For this review, take the finished solid that the model builds, in its own axes (mm). Face numbers are marked on the shaded views. A direction names the side the tool comes from. Coordinates: 2 decimals unless noted, no trailing zeros. Loops run counter-clockwise (first coordinate to the right, second up) from the corner with the lowest first, then second, coordinate; pieces in that order, holes last. Notation, with made-up numbers: (79.25, 87) -> (110.25, 87) arc R7 cw to (110.25, 95) -> close; hole circle Ø4 at (-7.75, -11.5). An arc over 180 degrees is marked (long way). One line per item, written item: value.
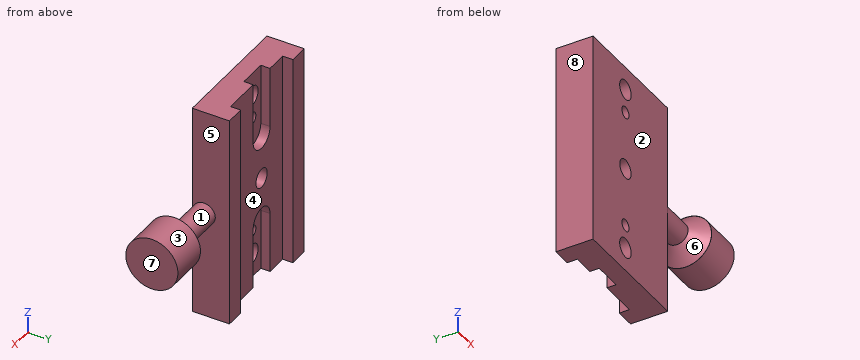
from build123d import *

# Parameters (mm, degrees)
BOSS_EXTRUDE1_DEPTH = 90
SKETCH2_R           = 4.75
BOSS_EXTRUDE2_DEPTH = 37
SKETCH3_R           = 11
BOSS_EXTRUDE3_DEPTH = 16
CHAMFER1_SIZE       = 6.2
SKETCH4_R           = 4
SKETCH4_R_2         = 2.5
SKETCH4_R_3         = 4.1
CUT_EXTRUDE1_DEPTH  = 16.97152885
CUT_EXTRUDE2_DEPTH  = 3.9


with BuildPart() as part:
    # Sketch1 → Boss-Extrude1 (new body)
    with BuildSketch(Plane.XY):
        Polygon((0, 0), (30, 0), (30, 15.7), (22, 15.7), (22, 11.4), (0, 11.4), (-15, 11.4), (-15, 15.7), (-23, 15.7), (-23, 0), align=None)
    extrude(amount=BOSS_EXTRUDE1_DEPTH)

    # Sketch2 → Boss-Extrude2 (add)
    with BuildSketch(Plane(origin=(30, 0, 0), x_dir=(0, 0, -1), z_dir=(1, 0, 0))):
        with Locations((-45, 4.97152885)):
            Circle(SKETCH2_R)
    extrude(amount=BOSS_EXTRUDE2_DEPTH)

    # Sketch3 → Boss-Extrude3 (add)
    with BuildSketch(Plane(origin=(67, 0, 0), x_dir=(0, 0, -1), z_dir=(1, 0, 0))):
        with Locations((-45, 4.97152885)):
            Circle(SKETCH3_R)
    extrude(amount=-BOSS_EXTRUDE3_DEPTH)

    # Chamfer1
    chamfer1_edges = [part.edges().sort_by_distance(p)[0] for p in [
        (51, 4.97152885, 49.75),
    ]]
    chamfer(chamfer1_edges, length=CHAMFER1_SIZE)

    # Sketch4 → Cut-Extrude1 (cut, through all)
    with BuildSketch(Plane(origin=(0, 0, 0), x_dir=(1, 0, 0), z_dir=(0, 1, 0))):
        with Locations((0, -45)):
            Circle(SKETCH4_R)
        with Locations((0, -20)):
            Circle(SKETCH4_R_2)
        with Locations((0, -70)):
            Circle(SKETCH4_R_2)
        with Locations((0, -10)):
            Circle(SKETCH4_R_3)
        with Locations((0, -80)):
            Circle(SKETCH4_R_3)
    extrude(amount=CUT_EXTRUDE1_DEPTH, mode=Mode.SUBTRACT)

    # Sketch5 → Cut-Extrude2 (cut)
    with BuildSketch(Plane(origin=(0, 11.4, 0), x_dir=(1, 0, 0), z_dir=(0, 1, 0))):
        with BuildLine():
            Line((-6, -25.72942469), (-6, 7.985784124))
            ThreePointArc((-6, 7.985784124), (0, 13.985784124), (6, 7.985784124))
            Line((6, 7.985784124), (6, -25.72942469))
            ThreePointArc((6, -25.72942469), (0, -31.72942469), (-6, -25.72942469))
        make_face()
        with BuildLine():
            Line((-6, -64.27057531), (-6, -97.985784124))
            ThreePointArc((-6, -97.985784124), (0, -103.985784124), (6, -97.985784124))
            Line((6, -97.985784124), (6, -64.27057531))
            ThreePointArc((6, -64.27057531), (0, -58.27057531), (-6, -64.27057531))
        make_face()
    extrude(amount=-CUT_EXTRUDE2_DEPTH, mode=Mode.SUBTRACT)


solid = part.part
1. Take a section at B-B, the plane x = 0. Give the boundary of the cut face in (y, z).
Return value:
outline: (0, 0) -> (7.5, 0) -> (7.5, 5.9) -> (0, 5.9) -> close; (0, 14.1) -> (7.5, 14.1) -> (7.5, 17.5) -> (0, 17.5) -> close; (0, 22.5) -> (7.5, 22.5) -> (7.5, 31.73) -> (11.4, 31.73) -> (11.4, 41) -> (0, 41) -> close; (0, 49) -> (11.4, 49) -> (11.4, 58.27) -> (7.5, 58.27) -> (7.5, 67.5) -> (0, 67.5) -> close; (0, 72.5) -> (7.5, 72.5) -> (7.5, 75.9) -> (0, 75.9) -> close; (0, 84.1) -> (7.5, 84.1) -> (7.5, 90) -> (0, 90) -> close
2. Take a section at A-A, the plane z = 20. Give the boundary of the cut face in (x, y).
Return value:
outline: (-23, 0) -> (-2.5, 0) -> (-2.5, 7.5) -> (-6, 7.5) -> (-6, 11.4) -> (-15, 11.4) -> (-15, 15.7) -> (-23, 15.7) -> close; (2.5, 0) -> (30, 0) -> (30, 15.7) -> (22, 15.7) -> (22, 11.4) -> (6, 11.4) -> (6, 7.5) -> (2.5, 7.5) -> close
3. Take a section at D-D, the plane x = 15. Give the boundary of the cut face in (y, z).
Return value:
outline: (0, 0) -> (11.4, 0) -> (11.4, 90) -> (0, 90) -> close
4. Take a section at C-C, the plane z = 80. Give the boundary of the cut face in (x, y).
Return value:
outline: (-23, 0) -> (-4.1, 0) -> (-4.1, 7.5) -> (-6, 7.5) -> (-6, 11.4) -> (-15, 11.4) -> (-15, 15.7) -> (-23, 15.7) -> close; (4.1, 0) -> (30, 0) -> (30, 15.7) -> (22, 15.7) -> (22, 11.4) -> (6, 11.4) -> (6, 7.5) -> (4.1, 7.5) -> close
5. To check wall thickness, follow probe 1 along Z at (x, y) = (0, 2.75); probe 2 along X at (y, z) = (2, 10); probe 3 along X at (y, z) = (10.25, 68). State the ranges of each line that lie inside material, in increasing order. Write a range as from..to.
Return value:
probe 1: z = 0..5.9, 14.1..17.5, 22.5..41, 49..67.5, 72.5..75.9, 84.1..90
probe 2: x = -23..-4.1, 4.1..30
probe 3: x = -23..-6, 6..30
6. The part is to be moulded in two halves that separate along X. For the marked faces 5, 6, 7 and 8, say which applies: pulls with the +X half, pulls with the -X half, needs draft (parallel to the pull), parting line crosses it, or undercut.
Return value:
face 5: undercut
face 6: undercut
face 7: pulls with the +X half
face 8: pulls with the -X half
7. Insertion check: pin 1 Ø4.5 at (y, z) = (9.5, 14.5) entering from +X; pin 2 Ø13 at (x, z) = (0, 80) entering from -Y; pin 3 Ø10.5 at (x, z) = (0, 10) entering from +Y. Each pin has a flat end and moves straight along its axis. Give the tip position at first contact, or say it passes through.
Return value:
pin 1: stops at x = 30
pin 2: stops at y = 0
pin 3: stops at y = 7.5
8. For the marked faces 1, 2, 3 and 4, list the 3-axis set-ups (+Z, -Z, +X, -X, +Y, -Y) from which the entire face can be reached by the end or side of a thin tool; tool diameter is ignored.
Return value:
face 1: none
face 2: +Z, -Z, -X, -Y
face 3: +X
face 4: +Z, -Z, +Y
